Read the model definition and answer for the solid it produces. Units are mm, in the model's axes. A direction names the side the tool comes from. Coordinates: 2 decimals unless noted, no trailing zeros. Loops run counter-clockwise (first coordinate to the right, second up) from the corner with the lowest first, then second, coordinate; pieces in that order, holes last.
from build123d import *

# Parameters (mm, degrees)
SKETCH1_R        = 6
PROBE_BODY_DEPTH = 70
SKETCH2_R        = 0.8
PIN_WELLS_DEPTH  = 3
CABLE_STUB_START = 70
SKETCH3_R        = 2
CABLE_STUB_DEPTH = 15


with BuildPart() as part:
    # Sketch1 → Probe_Body (new body)
    with BuildSketch(Plane(origin=(0, 0, 0), x_dir=(1, 0, 0), z_dir=(0, 1, 0))):
        with Locations(Location((0, 0, 0), (0, 0, 270))):
            Circle(SKETCH1_R)
    extrude(amount=PROBE_BODY_DEPTH)

    # Sketch2 → Pin_Wells (cut)
    with BuildSketch(Plane(origin=(0, 0, 0), x_dir=(1, 0, 0), z_dir=(0, 1, 0))):
        with Locations(Location((-2.5, 0, 0), (0, 0, 270))):
            Circle(SKETCH2_R)
        with Locations(Location((2.5, 0, 0), (0, 0, 270))):
            Circle(SKETCH2_R)
    extrude(amount=PIN_WELLS_DEPTH, mode=Mode.SUBTRACT)

    # Sketch3 → Cable_Stub (add)
    with BuildSketch(Plane(origin=(0, 0, 0), x_dir=(1, 0, 0), z_dir=(0, 1, 0)).offset(CABLE_STUB_START)):
        with Locations(Location((0, 0, 0), (0, 0, 270))):
            Circle(SKETCH3_R)
    extrude(amount=CABLE_STUB_DEPTH)


solid = part.part
Item 1: A cutting plane is placed at A-A on x = 0. Determine the outline of the cut face in (y, z).
Numbers:
outline: (0, -6) - (70, -6) - (70, -2) - (85, -2) - (85, 2) - (70, 2) - (70, 6) - (0, 6) - close
Item 2: Determine the mould class of faces 1 (the face through (0, 85, 0)), 2 (the face through (-3.28, 1.48, -0.17)), 3 (the face through (1.802, 34.51, 5.723)) for opening direction X: released by +X, released by -X, zero draft, split by the parting line, or undercut.
Numbers:
face 1: zero draft
face 2: undercut
face 3: split by the parting line
Item 3: A cutting plane is placed at D-D on y = 73.5. Determine the outline of the cut face in (x, z), then the cut area to 3 significant figures.
Numbers:
outline: circle Ø4 at (0, 0)
area: 12.6 mm2
Item 4: Which of the six approach directions +Z, -Z, +X, -X, +Y, -Y give full straight-line access (tool end or side, diameter ignored) to faces 4 (the face through (0, 0, 0)), 5 (the face through (1.72, 1.48, -0.17)), 6 (the face through (0, 70, 3))?
Numbers:
face 4: +Z, -Z, +X, -X, -Y
face 5: -Y
face 6: +Y
Item 5: A cutting plane is placed at C-C on y = 63.5. Determine the outline of the cut face in (x, z).
Numbers:
outline: circle Ø12 at (0, 0)
Item 6: Given pin 1 (3 mm diameter, centred on y = 28.5, z = -5, fed in from +X); pin 2 (0.8 mm diameter, centred on x = -2.5, z = 0, fed in from -Y); pin 3 (1 mm diameter, centred on y = 11, z = 1, fed in from -X), each flat-ended and moving along its own axis, determine where each tip first touches the part or whether it passes through.
Numbers:
pin 1: stops at x = 4.87
pin 2: stops at y = 3
pin 3: stops at x = -5.98
Item 7: Find the intervals of material crossed by line 1 along X through (y, z) = (1.2, 0); line 2 along Y through (x, z) = (2.5, -4.5); line 3 along Y through (x, z) = (-2.5, 0), in increasing order.
Numbers:
line 1: x = -6 to -3.3, -1.7 to 1.7, 3.3 to 6
line 2: y = 0 to 70
line 3: y = 3 to 70
Item 8: A cutting plane is placed at B-B on z = 0. Determine the outline of the cut face in (x, y).
Numbers:
outline: (-6, 0) - (-3.3, 0) - (-3.3, 3) - (-1.7, 3) - (-1.7, 0) - (1.7, 0) - (1.7, 3) - (3.3, 3) - (3.3, 0) - (6, 0) - (6, 70) - (2, 70) - (2, 85) - (-2, 85) - (-2, 70) - (-6, 70) - close
